Source: CAD feature listing. Evaluate the final solid. Frame: model axes, mm. Face numbers are marked on the shaded views. A direction names the side the tool comes from. Give positions to 0.01 mm unless a question says otherwise; leave off trailing zeros. Loops run counter-clockwise (first coordinate to the right, second up) from the corner with the lowest first, then second, coordinate; pieces in that order, holes last.
```python
from build123d import *

# Parameters (mm, degrees)
SKETCH1_R           = 70
BOSS_EXTRUDE1_DEPTH = 370
SKETCH4_R           = 10
BOSS_EXTRUDE2_DEPTH = 80
BOSS_EXTRUDE3_START = 100
SKETCH5_R           = 10
BOSS_EXTRUDE3_DEPTH = 100
CUT_EXTRUDE1_START  = -15
SKETCH6_R           = 10
CUT_EXTRUDE1_DEPTH  = 15
BOSS_EXTRUDE4_DEPTH = 25
SKETCH8_R           = 15
BOSS_EXTRUDE5_DEPTH = 535
BOSS_EXTRUDE7_DEPTH = 55
BOSS_EXTRUDE8_START = 55
SKETCH10_R          = 15
BOSS_EXTRUDE8_DEPTH = 55


with BuildPart() as part:
    # Sketch1 → Boss-Extrude1 (new body)
    with BuildSketch(Plane.XY):
        Circle(SKETCH1_R)
    extrude(amount=BOSS_EXTRUDE1_DEPTH)

    # Sketch4 → Boss-Extrude2 (add)
    with BuildSketch(Plane.XY.offset(370)):
        Circle(SKETCH4_R)
    extrude(amount=BOSS_EXTRUDE2_DEPTH)

    # Sketch5 → Boss-Extrude3 (add)
    with BuildSketch(Plane(origin=(0, 0, 0), x_dir=(-1, 0, 0), z_dir=(0, 0, -1)).offset(BOSS_EXTRUDE3_START)):
        with Locations(Location((0, 0, 0), (0, 0, 180))):
            Circle(SKETCH5_R)
    extrude(amount=-BOSS_EXTRUDE3_DEPTH)

    # Sketch6 → Cut-Extrude1 (cut)
    with BuildSketch(Plane.XY.offset(450).offset(CUT_EXTRUDE1_START)):
        Circle(SKETCH6_R)
    extrude(amount=CUT_EXTRUDE1_DEPTH, mode=Mode.SUBTRACT)

    # Sketch7 → Boss-Extrude4 (add)
    with BuildSketch(Plane(origin=(0, 0, -100), x_dir=(-1, 0, 0), z_dir=(0, 0, -1))):
        with BuildLine():
            Line((5, 8.660254038), (5, 12.820254038))
            Line((5, 12.820254038), (-5, 12.820254038))
            Line((-5, 12.820254038), (-5, 8.660254038))
            ThreePointArc((-5, 8.660254038), (0, 10), (5, 8.660254038))
        make_face()
    extrude(amount=-BOSS_EXTRUDE4_DEPTH)

    # Sketch8 → Boss-Extrude5 (add)
    with BuildSketch(Plane(origin=(0, 0, -100), x_dir=(-1, 0, 0), z_dir=(0, 0, -1))):
        Circle(SKETCH8_R)
    extrude(amount=-BOSS_EXTRUDE5_DEPTH)



with BuildPart() as body_2:
    # Sketch9 → Boss-Extrude7 (new body)
    with BuildSketch(Plane(origin=(0, 0, -100), x_dir=(-1, 0, 0), z_dir=(0, 0, -1))):
        with BuildLine():
            Line((-5, 14.142135624), (-5, 18.302135624))
            Line((-5, 18.302135624), (5, 18.302135624))
            Line((5, 18.302135624), (5, 14.142135624))
            ThreePointArc((5, 14.142135624), (0, 15), (-5, 14.142135624))
        make_face()
    extrude(amount=BOSS_EXTRUDE7_DEPTH)


with BuildPart() as part_1:
    add(part.part)

    add(body_2.part)  # Boss-Extrude8 merges body 2
    # Sketch10 → Boss-Extrude8 (add)
    with BuildSketch(Plane(origin=(0, 0, -100), x_dir=(-1, 0, 0), z_dir=(0, 0, -1)).offset(BOSS_EXTRUDE8_START)):
        with Locations(Location((0, 0, 0), (0, 0, 70.528779366))):
            Circle(SKETCH10_R)
    extrude(amount=-BOSS_EXTRUDE8_DEPTH)


solid = part_1.part
```
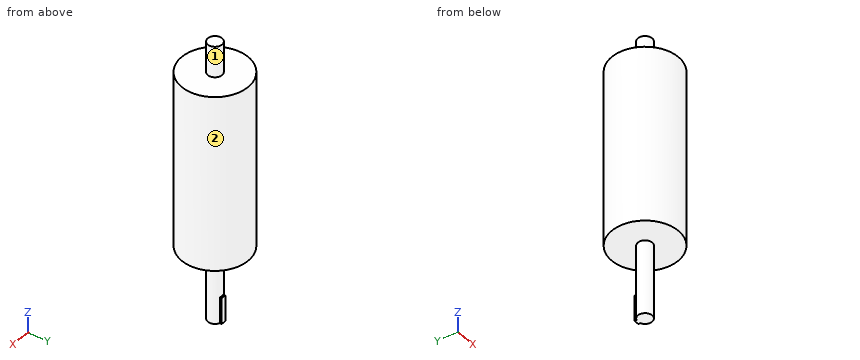
(1) Ray query, line 1 along X through (y, z) = (-2, 55); line 2 along Z through (x, y) = (-20, 53.5); line 3 along X through (y, z) = (0, -61). Return the intervals inside material, ascending.
A:
line 1: x = -69.97 to 69.97
line 2: z = 0 to 370
line 3: x = -15 to 15
(2) Section A-A, the plane x = 0. Return the cut outline in (y, z), then the cut area to 3 significant figures.
A:
outline: (-70, 0) - (-15, 0) - (-15, -155) - (18.3, -155) - (18.3, -100) - (15, -100) - (15, 0) - (70, 0) - (70, 370) - (15, 370) - (15, 435) - (-15, 435) - (-15, 370) - (-70, 370) - close
area: 58,600 mm2
(3) Section C-C, the plane y = -5. Return the cut outline in (x, z), then the cut area to 3 significant figures.
A:
outline: (-69.82, 0) - (-14.14, 0) - (-14.14, -155) - (14.14, -155) - (14.14, 0) - (69.82, 0) - (69.82, 370) - (14.14, 370) - (14.14, 435) - (-14.14, 435) - (-14.14, 370) - (-69.82, 370) - close
area: 57,900 mm2
(4) Section B-B, the plane z = -28. Return the cut outline in (x, y), then the cut area to 3 significant figures.
A:
outline: circle Ø30 at (0, 0)
area: 707 mm2
(5) First-contact query: pin 1 (8 mm diameter, centred on y = -32, z = 332, fed in from -X); pin 2 (2 mm diameter, centred on x = 0, y = 16.5, fed in from +Z); pin 3 (4 mm diameter, centred on y = 28.5, z = 107.5, fed in from +X). Flat tips, straight axial feed; report the tip coordinate or a pass-through.
A:
pin 1: stops at x = -64.16
pin 2: stops at z = 370
pin 3: stops at x = 64.79
(6) Section D-D, the plane z = 298. Return the cut outline in (x, y).
A:
outline: circle Ø140 at (0, 0)
(7) Reachability of the marked faces 1 and 2 from +Z, -Z, +X, -X, +Y, -Y: full face, straight path, thin tool, end or side. Return the list, or none.
A:
face 1: +Z
face 2: +Z, -Z
